```python
from build123d import *

# Parameters (mm, degrees)
F1_DEPTH = 21
F2_R     = 2.5
F3_DEPTH = 25
F4_R     = 2.5
F5_DEPTH = 25


with BuildPart() as f1:
    # F0 (on Top) → F1 (new body)
    with BuildSketch(Plane.XY):
        Polygon((0, 7), (0, 0), (7, 0), (7, 5.5), (13, 5.5), (13, 0), (20, 0), (20, 7), (14.5, 7), (14.5, 13), (20, 13), (20, 20), (13, 20), (13, 14.5), (7, 14.5), (7, 20), (0, 20), (0, 13), (5.5, 13), (5.5, 7), align=None)
    extrude(amount=F1_DEPTH)

    # F2 (on face) → F3 (cut)
    with BuildSketch(Plane.YZ.offset(14.5)):
        with Locations((10, 70)):
            Circle(F2_R)
    extrude(amount=-F3_DEPTH, mode=Mode.SUBTRACT)

    # F4 (on face) → F5 (cut)
    with BuildSketch(Plane.XZ.offset(-5.5)):
        with Locations((10, 70)):
            Circle(F4_R)
    extrude(amount=-F5_DEPTH, mode=Mode.SUBTRACT)


solid = f1.part
```
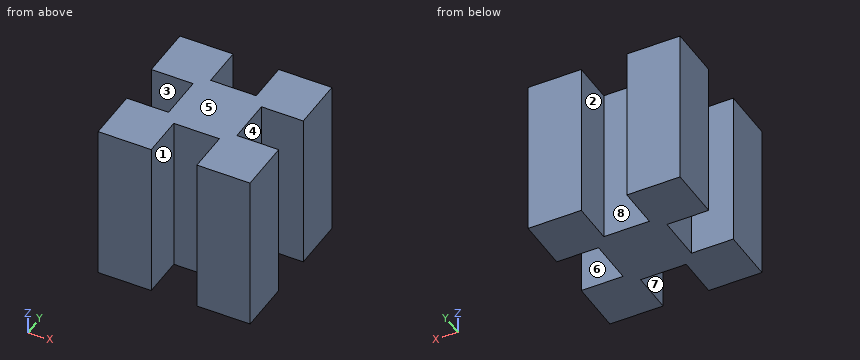
Design review of the part built by this model. Coordinates are the model's own, in mm. Face numbers are marked on the shaded views. A direction names the side the tool comes from. Round coordinates to 2 decimals unless told otherwise and drop trailing zeros. Order: outer loops, then holes, each group sorted by start corner. A loop starts at its lowest first (then second) coordinate and runs counter-clockwise, first axis right, second up. Notation, with made-up numbers: (-35.75, 68) - (-12.75, 68) arc R22 ccw to (-12.75, 88) - close; hole circle Ø9 at (31, -2). An arc over 180 degrees is marked (long way). Return JSON: item names as keys, results as strings.
Q1. Consider section D-D on x = 8. Write out the cut boundary in (y, z), plus the area to 3 significant figures.
Computed values:
{"outline": "(5.5, 0) - (14.5, 0) - (14.5, 21) - (5.5, 21) - close", "area": "189 mm2"}
Q2. Consider section C-C on z = 5.25. Write out the cut boundary in (x, y).
Computed values:
{"outline": "(0, 0) - (7, 0) - (7, 5.5) - (13, 5.5) - (13, 0) - (20, 0) - (20, 7) - (14.5, 7) - (14.5, 13) - (20, 13) - (20, 20) - (13, 20) - (13, 14.5) - (7, 14.5) - (7, 20) - (0, 20) - (0, 13) - (5.5, 13) - (5.5, 7) - (0, 7) - close"}
Q3. The part is to be moulded in two halves that separate along Y. For the marked faces 6, 7 and 8, say which applies: pulls with the +Y half, pulls with the -Y half, needs draft (parallel to the pull), parting line crosses it, or undercut.
Computed values:
{"face 6": "undercut", "face 7": "needs draft", "face 8": "pulls with the +Y half"}
Q4. For pin 1 Ø5 at (x, z) = (10, 6) entering from -Y; pin 2 Ø3 at (x, z) = (9, 13.5) entering from +Y, all flat-tipped, find the tip position at first contact; note any pin that passes through.
Computed values:
{"pin 1": "stops at y = 5.5", "pin 2": "stops at y = 14.5"}
Q5. Consider section A-A on y = 3.25. Write out the cut boundary in (x, z).
Computed values:
{"outline": "(0, 0) - (7, 0) - (7, 21) - (0, 21) - close; (13, 0) - (20, 0) - (20, 21) - (13, 21) - close"}
Q6. Machinability: for the marked faces 1, 2, 3, 4 and 5, which of the approach directions +Z, -Z, +X, -X, +Y, -Y give a long, thin tool a straight path to every point of the face, cutting with its end or side? Answer none if there is none.
Computed values:
{"face 1": "+Z, -Z, -Y", "face 2": "+Z, -Z, +Y", "face 3": "+Z, -Z, -X", "face 4": "+Z, -Z, +X", "face 5": "+Z, +X, -X, +Y, -Y"}
Q7. Wall thickness on L1, parallel to Y at x = 16.5, z = 10.75; L2, parallel to Y at x = 10, z = 1: over which ranges is each line inside the solid? List them lowest first. Write a range as [from, to].
Computed values:
{"L1": "y = [0, 7], [13, 20]", "L2": "y = [5.5, 14.5]"}
